Autodesk Inventor part; units mm, degrees
ref_plane "Work Plane1" through (-6.3375, 0, 0) normal (0, -0.8660254, -0.5) x (1, 0, 0)
ref_plane "YZ Plane" through (0, 0, 0) normal (1, 0, 0) x (0, 1, 0)
ref_plane "XZ Plane" through (0, 0, 0) normal (0, 1, 0) x (-1, 0, 0)
sketch "Sketch1" plane through (0, 0, 0) normal (1, 0, 0) x (0, 1, 0)
  line L0 (-3.1754, 0) -> (-1.5877, 2.75)
  line L1 (-1.5877, 2.75) -> (1.5877, 2.75)
  line L2 (1.5877, 2.75) -> (3.1754, 0)
  line L3 (3.1754, 0) -> (1.5877, -2.75)
  line L4 (1.5877, -2.75) -> (-1.5877, -2.75)
  line L5 (-1.5877, -2.75) -> (-3.1754, 0)
  point P0 (0, 0)
  point P1 (0, 0)
  dimension "d0" = 6.3509
extrude "Body" add sketch "Sketch1" along normal blind 2.4
sketch "Sketch2" plane through (0, 0, 0) normal (0, 0, 1) x (1, 0, 0)
  line L0 (0, 1.5877) -> (0, 3.1754)
  line L1 (0, 3.1754) -> (2.4, 3.1754)
  line L2 (2.4, 1.5877) -> (2.4, 3.1754)
  line L3 (-0.48, 0) -> (2.88, 0)
  line L4 (0.1984, 3.1754) -> (0, 2.75)
  line L5 (2.2016, 3.1754) -> (2.4, 2.75)
  dimension "d3" = 25
  dimension "d4" = 25
  dimension "d5" = 5.5
  dimension "d6" = 5.5
revolve "Chamfer1" cut sketch "Sketch2" angle 360 about axis through (-10, 0, 0) along (1, 0, 0)
sketch "Sketch3" plane through (2.4, 0, 0) normal (1, 0, 0) x (0, 0, -1)
  arc A0 (-1.375, -2.3816) -> (1.375, -2.3816) centre (0, 0) ccw
hole "Thread" at (2.4, 0, 0) direction (-1, 0, 0) diameter 2.459 end through all
chamfer "Chamfer2" distance 0.2706 angle 30 1 edges at (2.4, 0, 1.2295) measured on face at (2.4, -2.2301, -0.0494)
chamfer "Chamfer3" distance 0.2706 angle 30 1 edges at (0, 0, 1.2295) measured on face at (0, -2.2301, -0.0494)
ref_plane "Work Plane1" through (-6.3375, 0, 0) normal (0, -0.8660254, -0.5) x (1, 0, 0)
equation "\"d0\" = 1.1547 * SW"
equation "\"d1\" = KOH"
equation "\"d3\" = ANG1"
equation "\"d4\" = ANG2"
equation "\"d5\" = SW0"
equation "\"d6\" = SW01"
equation "\"d8\" = -0.5 * GD1 + 0.5 * NND"
equation "\"d40\" = -0.5 * GD1 + 0.5 * NND"
equation "\"d10\" = -0.5 * GD1 + 0.5 * NND"
equation "\"d41\" = -0.5 * GD1 + 0.5 * NND"
equation "\"ANG1\" = 25deg"
equation "\"ANG2\" = 25deg"
equation "\"NND\" = 3"
equation "\"KOH\" = 2.4"
equation "\"SW\" = 5.5"
equation "\"SW0\" = SW"
equation "\"SW01\" = SW"
equation "\"GUL\" = 0.541266 * PTC"
equation "\"THREADDIA\" = 3"
equation "\"TOA\" = 30deg"
equation "\"PTC\" = 0.5"
equation "\"E0\" = 1.155 * SW"
equation "\"GAL\" = 0.541266 * PTC"
equation "\"SD2\" = 0"
equation "\"WFT\" = 0"
properties part number "ANSI B 18.2.4.1 M - M3 x 0.5" material "Steel, Mild"
Could you check a few things on this model? Use its own coordinates, in mm. Round coordinates to 2 decimals unless told otherwise and drop trailing zeros. Write each loop counter-clockwise with the first axis right and the second up, starting at its lowest first coordinate (ties: lowest second). Pieces come first, ordered by that corner, then holes.
(1) If I drill on probe 1 along Z at (x, y) = (1.05, 0); probe 2 along Y at (x, z) = (0.25, -0.45); probe 3 along Z at (x, y) = (0.85, -0.5), over which ranges is the centre line in solid material (lowest first)?
Findings below:
probe 1: z = -2.75 to -1.23, 1.23 to 2.75
probe 2: y = -2.92 to -1.14, 1.14 to 2.92
probe 3: z = -2.75 to -1.12, 1.12 to 2.75
(2) For pin 1 (3 mm diameter, centred on y = -1, z = 0, fed in from +X), with a flat end and sliding along its axis, tell me the tip position at first contact or that it passes through.
Findings below:
pin 1: stops at x = 2.4
(3) Suppose I cut it at A-A on x = 1.35. Write out the boundary of the cut face in (y, z), and give its area (3 significant figures).
Findings below:
outline: (-3.18, 0) - (-1.59, -2.75) - (1.59, -2.75) - (3.18, 0) - (1.59, 2.75) - (-1.59, 2.75) - close; hole circle Ø2.46 at (0, 0)
area: 21.4 mm2
(4) Thinking about a two-plate mould opening in Y: for faces 1 (the face through (1.183, 2.37, 1.394)), 2 (the face through (1.185, 0.748, 0.976)), 3 (the face through (2.4, 1.2, -1.2)), which applies, +Y half, -Y half, draft (parallel to the pull), parting line (faces both ways), or undercut?
Findings below:
face 1: +Y half
face 2: undercut
face 3: draft
